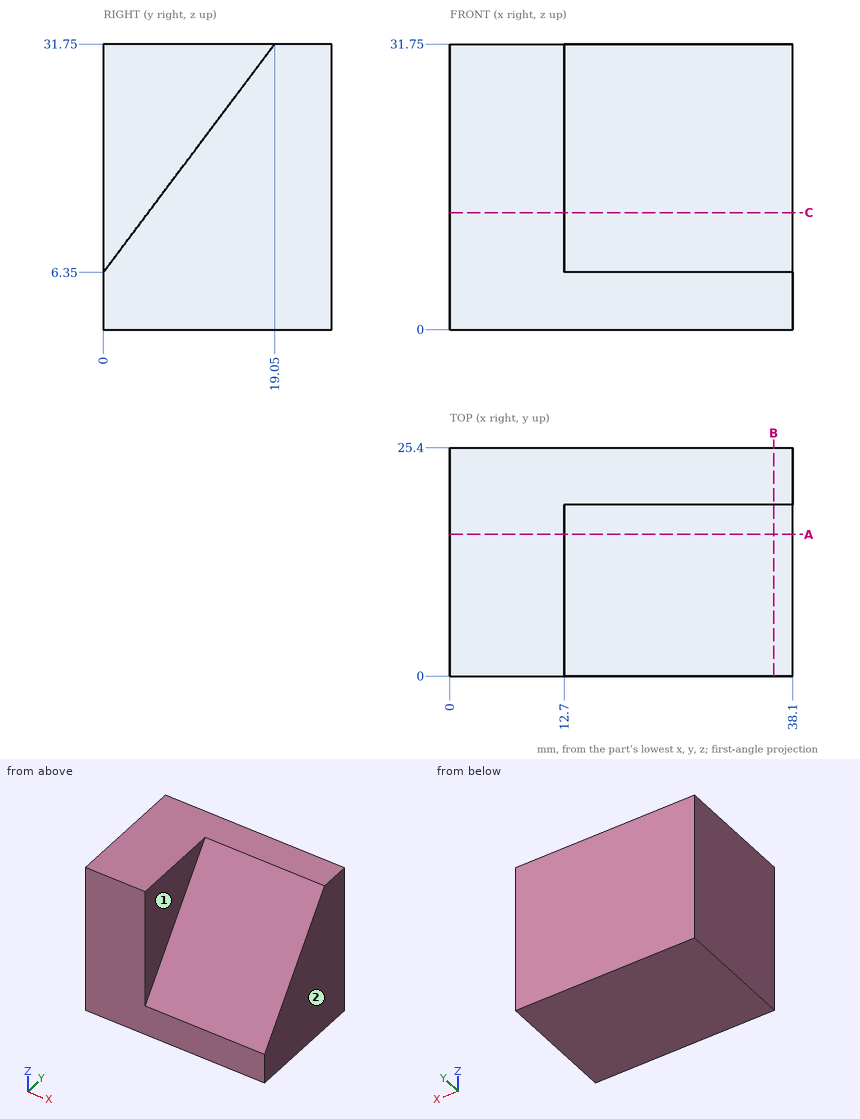
Can you work these out from the drawing? Everything is in mm from the part's minimum corner. A direction names the side the tool comes from. Give positions to 0.01 mm unless a question says otherwise; leave off trailing zeros. Order: outer loops, then holes, each group sorted by start corner. A loop starts at its lowest first (then second) coordinate and runs counter-clockwise, first axis right, second up.
Item 1: For the marked faces 1 and 2, which set-ups out of +Z, -Z, +X, -X, +Y, -Y let a thin tool reach every point of the face, with its end or its side?
Item 2: If we section it at B-B, the plane x = 36: Write out the boundary of the cut face in (y, z), plus the area to 3 significant figures.
Item 3: If we section it at A-A, the plane y = 15.75: Write out the boundary of the cut face in (x, z), plus the area to 3 significant figures.
Item 4: I need wall thicknesses on line 1 (X direction, y = 2.5, z = 14); line 2 (Z direction, x = 17, y = 18.5); line 3 (Y direction, x = 27, z = 29.5). Which ranges of each line are inside material? Lowest first, please.
Item 5: If we section it at C-C, the plane z = 13: Write out the boundary of the cut face in (x, y), plus the area to 3 significant figures.
Item 6: I'm going to push flat-ended pins straight in: pin 1 (2 mm diameter, centred on x = 29.5, y = 11.5, fed in from +Z); pin 2 (2 mm diameter, centred on y = 5, z = 18, fed in from +X); pin 3 (8 mm diameter, centred on x = 27, y = 7, fed in from +Z). Where does each tip first touch, or does it pass through?
Values:
1. face 1: +Z, +X, -Y
1. face 2: +Z, -Z, +X, +Y, -Y
2. outline: (0, 0) - (25.4, 0) - (25.4, 31.75) - (19.05, 31.75) - (0, 6.35) - close
2. area: 565 mm2
3. outline: (0, 0) - (38.1, 0) - (38.1, 27.35) - (12.7, 27.35) - (12.7, 31.75) - (0, 31.75) - close
3. area: 1,100 mm2
4. line 1: x = 0 to 12.7
4. line 2: z = 0 to 31.02
4. line 3: y = 17.36 to 25.4
5. outline: (0, 0) - (12.7, 0) - (12.7, 4.99) - (38.1, 4.99) - (38.1, 25.4) - (0, 25.4) - close
5. area: 841 mm2
6. pin 1: stops at z = 23.02
6. pin 2: stops at x = 12.7
6. pin 3: stops at z = 21.02
